```python
from build123d import *

# Parameters (mm, degrees)
F0_R     = 1.25
F1_DEPTH = 11.5


with BuildPart() as f1:
    # F0 (on Top) → F1 (new body)
    with BuildSketch(Plane.XY):
        with BuildLine():
            Line((-2, -34.75), (4.75, -34.75))
            Line((4.75, -34.75), (9.5, -34.75))
            Line((9.5, -34.75), (9.5, -27.75))
            Line((9.5, -27.75), (9.5, -11.459255))
            ThreePointArc((9.5, -11.459255), (9.824846, -10.10148), (10.729036, -9.03775))
            Line((10.729036, -9.03775), (16.25, -5))
            Line((16.25, -5), (16.25, -1.85))
            Line((16.25, -1.85), (13.6, -1.85))
            Line((13.6, -1.85), (13.6, 1.25))
            Line((13.6, 1.25), (16.25, 1.25))
            Line((16.25, 1.25), (16.25, 4.35))
            Line((16.25, 4.35), (13.6, 4.35))
            Line((13.6, 4.35), (13.6, 7.45))
            Line((13.6, 7.45), (16.25, 7.45))
            Line((16.25, 7.45), (16.25, 10.55))
            Line((16.25, 10.55), (13.6, 10.55))
            Line((13.6, 10.55), (13.6, 13.65))
            Line((13.6, 13.65), (16.25, 13.65))
            Line((16.25, 13.65), (16.25, 24.75))
            ThreePointArc((16.25, 24.75), (13.321068, 31.821068), (6.25, 34.75))
            Line((6.25, 34.75), (-13.841292, 34.75))
            Line((-13.841292, 34.75), (-13.841292, 31.442884))
            Line((-13.841292, 31.442884), (-16.25, 31.442884))
            Line((-16.25, 31.442884), (-16.25, 15.85))
            ThreePointArc((-16.25, 15.85), (-15.37132, 13.72868), (-13.25, 12.85))
            Line((-13.25, 12.85), (-5.433433, 12.85))
            Line((-5.433433, 12.85), (-5.433433, 17.35))
            Line((-5.433433, 17.35), (-8.25, 17.35))
            ThreePointArc((-8.25, 17.35), (-10.37132, 18.22868), (-11.25, 20.35))
            Line((-11.25, 20.35), (-11.25, 24.5))
            ThreePointArc((-11.25, 24.5), (-10.37132, 26.62132), (-8.25, 27.5))
            Line((-8.25, 27.5), (-0.5, 27.5))
            ThreePointArc((-0.5, 27.5), (6.571068, 24.571068), (9.5, 17.5))
            Line((9.5, 17.5), (9.5, -2.963436))
            Line((9.5, -2.963436), (4.008641, -6.877843))
            ThreePointArc((4.008641, -6.877843), (3.083159, -7.946693), (2.75, -9.320724))
            Line((2.75, -9.320724), (2.75, -9.936604))
            Line((2.75, -9.936604), (2.75, -27.75))
            Line((2.75, -27.75), (-2, -27.75))
            Line((-2, -27.75), (-2, -34.75))
        make_face()
        with Locations((0.375, -31.25)):
            Circle(F0_R, mode=Mode.SUBTRACT)
    extrude(amount=F1_DEPTH)


solid = f1.part
```
Source: CAD feature listing. Evaluate the final solid. Frame: model axes, mm. A direction names the side the tool comes from. Coordinates: 2 decimals unless noted, no trailing zeros. Order: outer loops, then holes, each group sorted by start corner. A loop starts at its lowest first (then second) coordinate and runs counter-clockwise, first axis right, second up. Notation, with made-up numbers: (80, 62.25) - (118, 62.25) arc R32 cw to (118, 100.25) - close; hole circle Ø4 at (72, 29). An arc over 180 degrees is marked (long way). One line per item, written item: value.
1) Cut plane B-B on x = -7. Output: boundary loops of the cut face in (y, z), plus the area to 3 significant figures.
Computed values:
outline: (12.85, 0) - (17.35, 0) - (17.35, 11.5) - (12.85, 11.5) - close; (27.5, 0) - (34.75, 0) - (34.75, 11.5) - (27.5, 11.5) - close
area: 135 mm^2
2) Cut plane C-C on y = -10.5. Output: boundary loops of the cut face in (x, z).
Computed values:
outline: (2.75, 0) - (9.66, 0) - (9.66, 11.5) - (2.75, 11.5) - close
3) Cut plane A-A on y = -31.25. Output: boundary loops of the cut face in (x, z) (3 decimals).
Computed values:
outline: (-2, 0) - (-0.875, 0) - (-0.875, 11.5) - (-2, 11.5) - close; (1.625, 0) - (9.5, 0) - (9.5, 11.5) - (1.625, 11.5) - close
4) Contact query for flat-ended pins moving along their axis: pin 1 (6 mm diameter, centred on y = -20, z = 7, fed in from -X); pin 2 (3 mm diameter, centred on y = -2, z = 1.5, fed in from -X); pin 3 (4 mm diameter, centred on y = -5, z = 4, fed in from -X); pin 4 (5 mm diameter, centred on x = -4, z = 10, fed in from -Y). Output: stop coordinate, or through.
Computed values:
pin 1: stops at x = 2.75
pin 2: stops at x = 8.75
pin 3: stops at x = 3.85
pin 4: stops at y = -34.75
5) Mould query, pull axis X, two halves, no side actions, for faces 6 (the face through (15, 13.65, 6)), 7 (the face through (13.6, 6, 6)), 8 (the face through (-5.433, 15, 6)). Classes: released by +X, released by -X, zero draft, split by the parting line, or undercut.
Computed values:
face 6: zero draft
face 7: released by +X
face 8: undercut
6) Ray query, line 1 (Y direction, x = -7.5, z = 6.25); line 2 (Y direction, x = 0.5, z = 10.75); line 3 (Y direction, x = -1, z = 1). Return the intervals inside material, ascending. Write a range as [from, to].
Computed values:
line 1: y = [12.85, 17.35], [27.5, 34.75]
line 2: y = [-34.75, -32.49], [-30.01, -27.75], [27.45, 34.75]
line 3: y = [-34.75, -27.75], [27.5, 34.75]
7) Reachability of faces 1 (the face through (-10.35, 18.21, 5.67)), 2 (the face through (-9, 12.85, 6)), 3 (the face through (0, -27.75, 6)), 4 (the face through (15, 10.55, 6)), 5 (the face through (13.45, -7.05, 5.67)) from +Z, -Z, +X, -X, +Y, -Y: full face, straight path, thin tool, end or side. Return the list, or none.
Computed values:
face 1: +Z, -Z
face 2: +Z, -Z, -X, -Y
face 3: +Z, -Z, -X
face 4: +Z, -Z, +X
face 5: +Z, -Z, +X, -Y
